Answer from the drawing. Dimensions are ordinates in mm from the lowest x, y and z of the part. A direction names the side the tool comes from. Round coordinates to 2 decimals unless told otherwise and drop trailing zeros. Write each loop counter-clockwise with the first axis right and the second up, starting at its lowest first coordinate (ties: lowest second). Pieces come first, ordered by that corner, then holes. Notation, with made-up numbers: (-35.75, -31) -> (-23.75, -31) arc R24 cw to (-23.75, -1) -> close; hole circle Ø8 at (19, -17.5). An arc over 180 degrees is marked (long way). Answer as a JSON object with one key per item and string values. Group by question number.
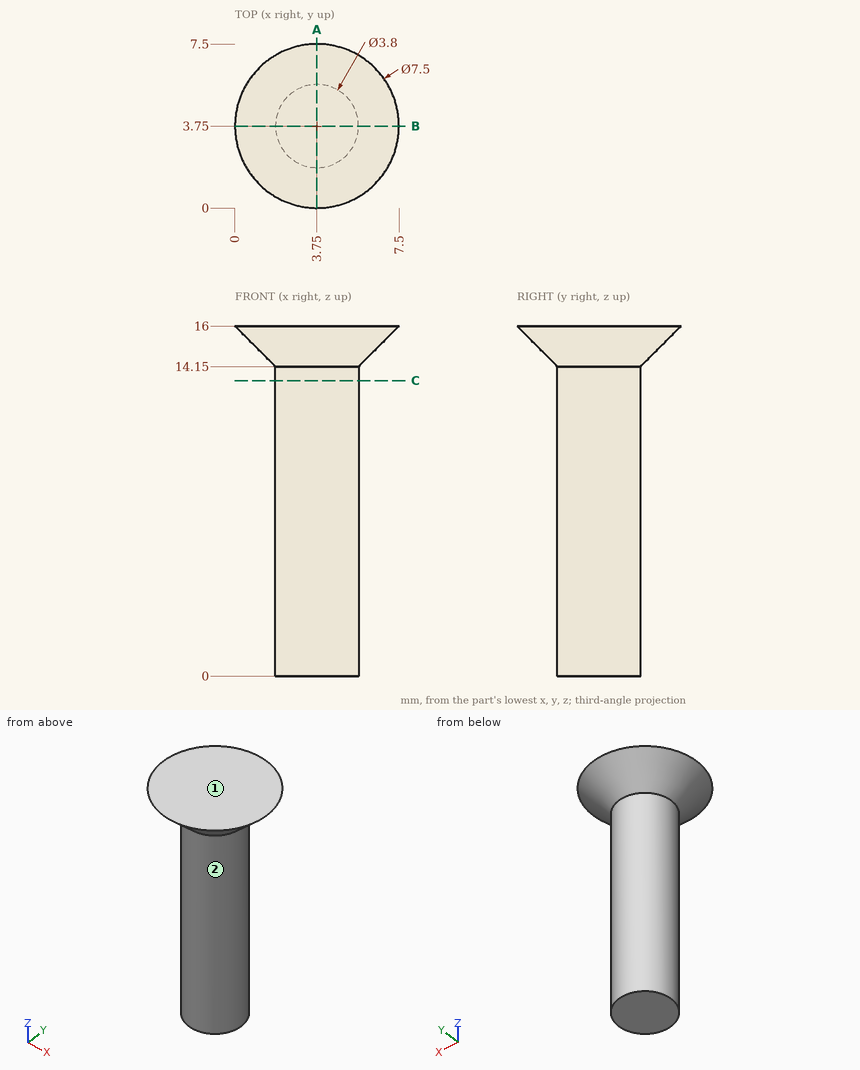
1) Straight lines are drawn through the part: L1, parallel to Y at x = 2.5, z = 15; L2, parallel to Z at x = 4.5, y = 0.75; L3, parallel to Y at x = 2.5, z = 3.25. For each, find the intervals that lie inside material, in ascending order.
2) A tool of negligible diameter and unlimited length cuts with its end or side. For the marked faces 1 and 2, from which of +Z, -Z, +X, -X, +Y, -Y can it reach the whole face along a straight path? Write none if from no direction.
3) A cutting plane is placed at A-A on x = 3.75. Determine the outline of the cut face in (y, z).
4) Each of these flat-tipped pins is pushed along its axis until it touches: P1, Ø2, axis at x = 6, z = 8.5, coming from the +Y side; P2, Ø1.5, axis at y = 3.5, z = 9.5, coming from the +X side. Where does it stop, or does it pass through?
5) A cutting plane is placed at C-C on z = 13.5. Determine the outline of the cut face in (x, y), plus the area to 3 significant figures.
Established:
{
 "1": {"L1": "y = 1.3 to 6.2", "L2": "z = 15.34 to 16", "L3": "y = 2.32 to 5.18"},
 "2": {"face 1": "+Z, +X, -X, +Y, -Y", "face 2": "-Z"},
 "3": {"outline": "(0, 16) -> (1.85, 14.15) -> (1.85, 0) -> (5.65, 0) -> (5.65, 14.15) -> (7.5, 16) -> close"},
 "4": {"P1": "stops at y = 5.18", "P2": "stops at x = 5.65"},
 "5": {"outline": "circle Ø3.8 at (3.75, 3.75)", "area": "11.3 mm²"}
}
